Read the model definition and answer for the solid it produces. Units are mm, in the model's axes. A direction names the side the tool comes from. Round coordinates to 2 decimals unless told otherwise and drop trailing zeros. Order: outer loops, then holes, each group sorted by start corner. A loop starts at its lowest first (then second) coordinate and runs counter-clockwise, first axis right, second up. Notation, with made-up numbers: (32.5, -20.5) - (76.5, -20.5) arc R19 cw to (76.5, -3.5) - close; hole circle Ø3 at (-22.5, 41). An arc over 180 degrees is marked (long way). Answer as a JSON object with one key per item and string values. Group by question number.
Q1. A cutting plane is placed at C-C on x = -78. Determine the outline of the cut face in (y, z), and give its area (3 significant figures).
Q2. Consider line 1 (X direction, y = 162.5, z = 382.5); line 2 (Y direction, x = -41, z = 596); line 3 (X direction, y = -21, z = 189). Determine where each line is inside the solid, lowest interval first.
Q3. A cutting plane is placed at A-A on y = -44.5. Determine the outline of the cut face in (x, z).
Q4. Given pin 1 Ø3 at (x, z) = (117.5, 882) entering from +Y; pin 2 Ø6 at (x, z) = (-94.5, 673) entering from -Y, each flat-ended and moving along its own axis, determine where each tip first touches the part or whether it passes through.
Q5. A cutting plane is placed at B-B on z = 619. Determine the outline of the cut face in (x, y).
Q6. A tool of negligible diameter and unlimited length cuts with its end or side. For faces 4 (the cylindrical face through (154.16, 16.22, 507)), 5 (the flat face through (173, -185, 493)), 6 (the flat face through (-2, -9, 493)), from which of +Z, -Z, +X, -X, +Y, -Y can it reach the whole face along a straight path? Write none if from no direction.
Q7. The mould has two halves that part along X. Classify faces 1 (the flat face through (185, -3, 493)), 2 (the flat face through (161, -106, 493)), 3 (the flat face through (173, 185, 493)): pulls with the +X half, pulls with the -X half, needs draft (parallel to the pull), parting line crosses it, or undercut.
```python
from build123d import *

# Parameters (mm, degrees)
F1_DEPTH = 1000
F2_R     = 24
F3_R     = 3


with BuildPart() as f1:
    # F0 (on Top) → F1 (new body)
    with BuildSketch(Plane.XY):
        Polygon((185, -185), (185, 185), (161, 185), (161, 9), (-161, 9), (-161, 185), (-185, 185), (-185, -185), (-161, -185), (-161, -9), (161, -9), (161, -185), align=None)
    extrude(amount=F1_DEPTH)

    # F2
    f2_edges = [f1.edges().sort_by_distance(p)[0] for p in [
        (-161, -9, 500),
        (161, -9, 500),
        (161, 9, 500),
        (-161, 9, 500),
    ]]
    fillet(f2_edges, radius=F2_R)

    # F3
    f3_edges = [f1.edges().sort_by_distance(p)[0] for p in [
        (161, 185, 500),
        (185, 185, 500),
        (-161, 185, 500),
        (-185, 185, 500),
        (185, -185, 500),
        (161, -185, 500),
        (-185, -185, 500),
        (-161, -185, 500),
    ]]
    fillet(f3_edges, radius=F3_R)


solid = f1.part
```
Result set:
{
 "1": {"outline": "(-9, 0) - (9, 0) - (9, 1000) - (-9, 1000) - close", "area": "18,000 mm²"},
 "2": {"line 1": "x = -185 to -161, 161 to 185", "line 2": "y = -9 to 9", "line 3": "x = -185 to -157.78, 157.78 to 185"},
 "3": {"outline": "(-185, 0) - (-161, 0) - (-161, 1000) - (-185, 1000) - close; (161, 0) - (185, 0) - (185, 1000) - (161, 1000) - close"},
 "4": {"pin 1": "stops at y = 9", "pin 2": "stops at y = -9"},
 "5": {"outline": "(-185, -182) arc R3 ccw to (-182, -185) - (-164, -185) arc R3 ccw to (-161, -182) - (-161, -33) arc R24 cw to (-137, -9) - (137, -9) arc R24 cw to (161, -33) - (161, -182) arc R3 ccw to (164, -185) - (182, -185) arc R3 ccw to (185, -182) - (185, 182) arc R3 ccw to (182, 185) - (164, 185) arc R3 ccw to (161, 182) - (161, 33) arc R24 cw to (137, 9) - (-137, 9) arc R24 cw to (-161, 33) - (-161, 182) arc R3 ccw to (-164, 185) - (-182, 185) arc R3 ccw to (-185, 182) - close"},
 "6": {"face 4": "+Z, -Z, +Y", "face 5": "+Z, -Z, +X, -X, -Y", "face 6": "+Z, -Z, -Y"},
 "7": {"face 1": "pulls with the +X half", "face 2": "undercut", "face 3": "needs draft"}
}
